from build123d import *

# Parameters (mm, degrees)
F0_W     = 25.4
F0_H     = 203.2
F1_DEPTH = 5.715
F2_W     = 4.3815
F2_H     = 203.2
F3_DEPTH = 4.445
F4_W     = 22.456064
F4_H     = 239.023939
F5_DEPTH = 2.0828
F6_R     = 1.778
F7_DEPTH = 25.4


with BuildPart() as f1:
    # F0 (on Top) → F1 (new body)
    with BuildSketch(Plane.XY):
        with Locations((12.7, 101.6)):
            Rectangle(F0_W, F0_H)
    extrude(amount=F1_DEPTH)

    # F2 (on face) → F3 (cut)
    with BuildSketch(Plane.XY.offset(5.715)):
        with Locations((19.39925, 101.6)):
            Rectangle(F2_W, F2_H)
    extrude(amount=-F3_DEPTH, mode=Mode.SUBTRACT)

    # F4 (on face) → F5 (cut)
    with BuildSketch(Plane.XY.offset(5.715)):
        with Locations((30.91247, 90.933911)):
            Rectangle(F4_W, F4_H)
    extrude(amount=-F5_DEPTH, mode=Mode.SUBTRACT)

    # F6 (on face) → F7 (cut)
    with BuildSketch(Plane.XY.offset(5.715)):
        with Locations((12.1285, 37.465)):
            Circle(F6_R)
        with Locations((12.1285, 10.16)):
            Circle(F6_R)
        with Locations((12.1285, 48.895)):
            Circle(F6_R)
        with Locations((12.1285, 87.63)):
            Circle(F6_R)
        with Locations((12.1285, 76.2)):
            Circle(F6_R)
        with Locations((12.1285, 114.808)):
            Circle(F6_R)
        with Locations((12.1285, 126.238)):
            Circle(F6_R)
        with Locations((12.1285, 153.416)):
            Circle(F6_R)
        with Locations((12.1285, 164.846)):
            Circle(F6_R)
        with Locations((12.1285, 192.024)):
            Circle(F6_R)
    extrude(amount=-F7_DEPTH, mode=Mode.SUBTRACT)


solid = f1.part
CAD build for the part. Positions are in the model's coordinates, mm. A direction names the side the tool comes from. Round coordinates to 2 decimals unless told otherwise and drop trailing zeros. Write each loop counter-clockwise with the first axis right and the second up, starting at its lowest first coordinate (ties: lowest second). Pieces come first, ordered by that corner, then holes. Notation, with made-up numbers: M 18.25,17 L 36.25,17 A10 ccw 36.25,36 Z; hole C 64,21.25 d8. An arc over 180 degrees is marked long. Put each result on its own line as item: value. Start each with the question number.
1) Saw through at C-C, the plane y = 63.5. Write the cut outline in (x, z) (1 decimal).
2) Pull direction Y, two halves, no side cores. Call faces 1 (the flat face through (10, 0, 3)), 2 (the flat face through (10, 203.2, 3)), 3 (the cylindrical face through (11.74, 151.68, 2.9)), 4 (the flat face through (25.4, 100, 2)): pulls with the +Y half, pulls with the -Y half, needs draft (parallel to the pull), parting line crosses it, or undercut.
3) Drill centre lines: probe 1 along X at (y, z) = (139, 3.4); probe 2 along X at (y, z) = (125, 1.3); probe 3 along Z at (x, y) = (20.5, 133). Where is each one in solid material? Low to high. Write a range as [from, to].
4) Saw through at B-B, the plane z = 4.55. Count the separate pieces of the cut face and the enclosed holes in it, and give its area (3 significant figures).
5) Saw through at A-A, the plane y = 10.16. Write the cut outline in (x, z) (1 decimal), and give its area (3 significant figures).
6) Pin check, flat tip, straight feed: pin 1 Ø1.1 at (x, y) = (23, 71) entering from +Z. Stop position of the tip, or through.
7) 3-axis set-ups, long thin cutter, end or side, ignore diameter. For faces 5 (the cylindrical face through (11.743, 85.894, 2.898)), 6 (the flat face through (23, 103, 3.632)), 7 (the flat face through (17.208, 100, 4)): which of +Z, -Z, +X, -X, +Y, -Y reach the whole face in a straight line?
Resolved:
1. outline: M 0,0 L 25.4,0 L 25.4,3.6 L 21.6,3.6 L 21.6,1.3 L 17.2,1.3 L 17.2,5.7 L 0,5.7 Z
2. face 1: pulls with the -Y half
2. face 2: pulls with the +Y half
2. face 3: undercut
2. face 4: needs draft
3. probe 1: [0, 17.21], [21.59, 25.4]
3. probe 2: [0, 10.85], [13.4, 17.21], [21.59, 25.4]
3. probe 3: [0, 1.27]
4. separate pieces: 1
4. enclosed holes: 10
4. area: 3,400 mm²
5. outline: M 0,0 L 10.4,0 L 10.4,5.7 L 0,5.7 Z; M 13.9,0 L 25.4,0 L 25.4,3.6 L 21.6,3.6 L 21.6,1.3 L 17.2,1.3 L 17.2,5.7 L 13.9,5.7 Z
5. area: 97.4 mm²
6. pin 1: z = 3.63
7. face 5: +Z, -Z
7. face 6: +Z, +X, +Y, -Y
7. face 7: +Z, +Y, -Y
